```python
from build123d import *

# Parameters (mm, degrees)
F3_DEPTH = 895
F4_R     = 6
F5_DEPTH = 50
F6_W     = 76
F6_H     = 90
F7_DEPTH = 5
F8_W     = 40
F8_H     = 60
F9_DEPTH = 935


with BuildPart() as f3:
    # F2 (on Right) → F3 (new body, symmetric)
    with BuildSketch(Plane.YZ):
        Polygon((-40, 75), (-40, -75), (40, -75), (40, 15), (0, 15), (0, 75), align=None)
    extrude(amount=F3_DEPTH, both=True)

    # F4 (on face) → F5 (cut)
    with BuildSketch(Plane(origin=(0, 40, 0), x_dir=(-1, 0, 0), z_dir=(0, 1, 0))):
        with Locations((-865, -45)):
            Circle(F4_R)
        with Locations((-845, -5)):
            Circle(F4_R)
        with Locations((845, -5)):
            Circle(F4_R)
        with Locations((865, -45)):
            Circle(F4_R)
    extrude(amount=-F5_DEPTH, mode=Mode.SUBTRACT)

    # F6 (on face) → F7 (cut)
    with BuildSketch(Plane(origin=(0, 40, 0), x_dir=(-1, 0, 0), z_dir=(0, 1, 0))):
        with Locations((-857, -30)):
            Rectangle(F6_W, F6_H)
        with Locations((857, -30)):
            Rectangle(F6_W, F6_H)
    extrude(amount=-F7_DEPTH, mode=Mode.SUBTRACT)

    # F8 (on Right) → F9 (join, symmetric)
    with BuildSketch(Plane.YZ):
        with Locations((-20, 45)):
            Rectangle(F8_W, F8_H)
    extrude(amount=F9_DEPTH, both=True)


solid = f3.part
```
Could you check a few things on this model? Use its own coordinates, in mm. A direction names the side the tool comes from. Coordinates: 2 decimals unless noted, no trailing zeros. Order: outer loops, then holes, each group sorted by start corner. A loop starts at its lowest first (then second) coordinate and runs counter-clockwise, first axis right, second up. Notation, with made-up numbers: M 15.5,57 L 50.5,57 A9 cw 50.5,74 Z; hole C 38,-9.75 d6. An arc over 180 degrees is marked long. Use a Markdown table: item, result. Add a question column.
Q1. If I drill on L1, parallel to Z at x = -865, y = 7.5; L2, parallel to Z at x = -845, y = 12.5; L3, parallel to Y at x = -831, z = -23.5, over which ranges is the centre line in solid material (lowest first)?
Q2. I want a section at B-B on x = -598. List the corners of the cut face in (y, z) for me.
Q3. I want a section at A-A on y = 15.5. List the corners of the cut face in (x, z) for me, then the cut area to 3 significant figures.
Q4. I'm going to push flat-ended pins straight in: pin 1 (1.5 mm diameter, centred on y = 36.5, z = -51.5, fed in from -X); pin 2 (1.5 mm diameter, centred on y = -30, z = -20.5, fed in from -X); pin 3 (20 mm diameter, centred on x = 913.5, y = -20, fed in from -Z). Where does each tip first touch, or does it pass through?
Q5. Which directions (+Z, -Z, +X, -X, +Y, -Y) give clear straight access to the entire face, cutting with the end or side of a thin tool? Please do faces 1 (the flat face through (-915, -20, 15)), 2 (the flat face through (895, -3, -29)), 3 (the flat face through (858, 35, -29)).
Checked values:
| question | item | result |
|---|---|---|
| 1 | L1 | -75 to -51, -39 to 15 |
| 1 | L2 | -75 to -11, 1 to 15 |
| 1 | L3 | -40 to 35 |
| 2 | outline | M -40,-75 L 40,-75 L 40,15 L 0,15 L 0,75 L -40,75 Z |
| 3 | outline | M -895,-75 L 895,-75 L 895,15 L -895,15 Z; hole C -865,-45 d12; hole C -845,-5 d12; hole C 845,-5 d12; hole C 865,-45 d12 |
| 3 | area | 161,000 mm² |
| 4 | pin 1 | x = -819 |
| 4 | pin 2 | x = -895 |
| 4 | pin 3 | z = 15 |
| 5 | face 1 | -Z, -X, +Y, -Y |
| 5 | face 2 | -Z, +X, +Y, -Y |
| 5 | face 3 | +Z, -Z, +X, +Y |
